Design review of the part shown in the three views and the two pictorial views. Dimensions are in mm from the part's minimum x, y and z. A direction names the side the tool comes from. Round coordinates to 2 decimals unless told otherwise and drop trailing zeros. Loops run counter-clockwise (first coordinate to the right, second up) from the corner with the lowest first, then second, coordinate; pieces in that order, holes last. Notation, with made-up numbers: (24, 76) -> (31, 76) arc R28 cw to (31, 103) -> close; hole circle Ø6 at (-28.5, 0). An arc over 180 degrees is marked (long way). Return JSON: item names as keys, results as strings. Group by question number.
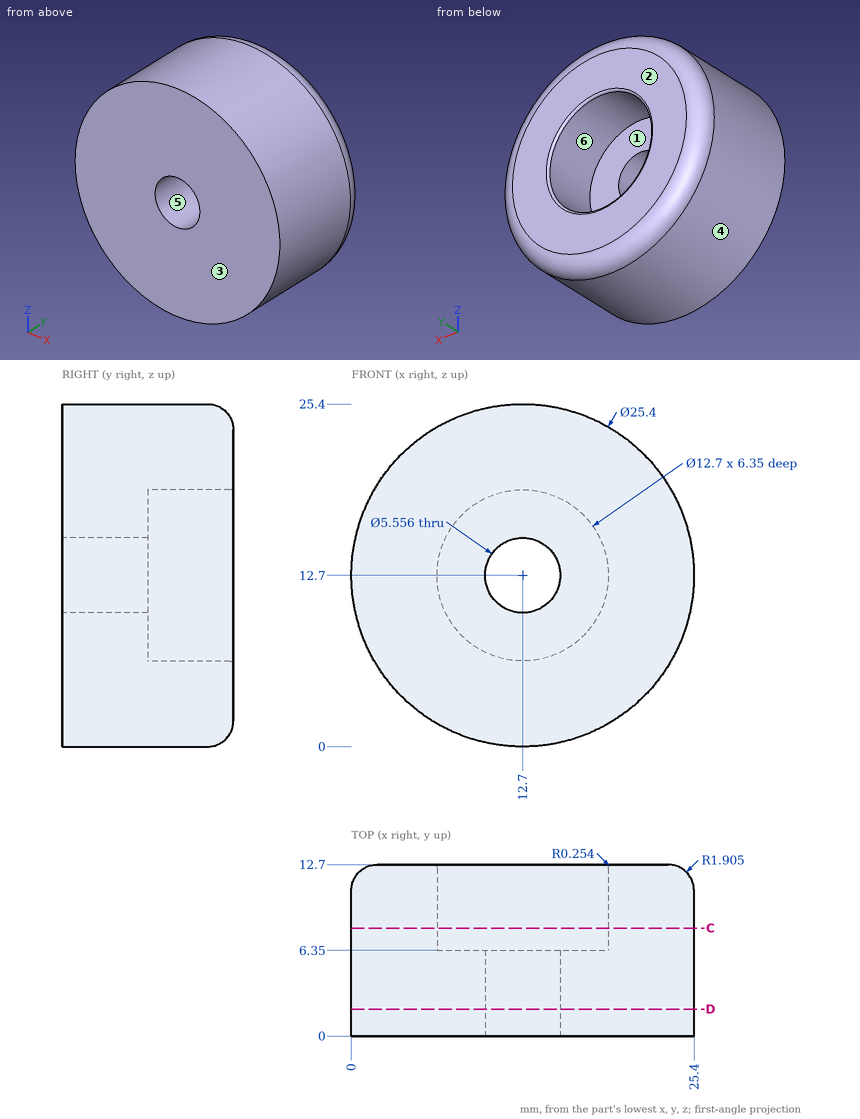
1. We need section D-D, the plane y = 2. Write out the cut boundary in (x, z).
2. For P1, Ø4, axis at x = 12.5, z = 9.5, coming from the +Y side; P2, Ø1, axis at x = 7, z = 6.5, coming from the -Y side; P3, Ø1, axis at y = 6, z = 16.5, coming from the +X side; P4, Ø4, axis at y = 7.5, z = 8.5, coming from the -X side, all flat-tipped, find the tip position at first contact; note any pin that passes through.
3. Wall thickness on line 1 (Z direction, x = 12.7, y = 5.25); line 2 (X direction, y = 9.25, z = 12.5): over which ranges is each line inside the solid? List them lowest first.
4. Tool access review of the marked faces 1 and 2: name each direction out of +Z, -Z, +X, -X, +Y, -Y from which nothing blocks a thin tool from reaching the whole face with its end or side.
5. We need section C-C, the plane y = 8. Write out the cut boundary in (x, z), then the cut area to 3 significant figures.
6. Draft analysis for pull direction X (two halves, no side actions). For the marked faces 3, 4, 5 and 6, state which applies: pulls with the +X half, pulls with the -X half, needs draft (parallel to the pull), parting line crosses it, or undercut.
Check sheet entries:
{
 "1": {"outline": "circle Ø25.4 at (12.7, 12.7); hole circle Ø5.56 at (12.7, 12.7)"},
 "2": {"P1": "stops at y = 6.35", "P2": "stops at y = 0", "P3": "stops at x = 24.96", "P4": "stops at x = 0.19"},
 "3": {"line 1": "z = 0 to 9.92, 15.48 to 25.4", "line 2": "x = 0 to 6.35, 19.05 to 25.4"},
 "4": {"face 1": "+Y", "face 2": "+Z, -Z, +X, -X, +Y"},
 "5": {"outline": "circle Ø25.4 at (12.7, 12.7); hole circle Ø12.7 at (12.7, 12.7)", "area": "380 mm²"},
 "6": {"face 3": "needs draft", "face 4": "parting line crosses it", "face 5": "undercut", "face 6": "undercut"}
}
